```python
from build123d import *

# Parameters (mm, degrees)
BOSS_EXTRUDE1_DEPTH     = 14
SKETCH2_R               = 2.9
CUT_EXTRUDE1_DEPTH      = 48
CUT_EXTRUDE2_DEPTH      = 10
SKETCH6_R               = 10.5
CUT_EXTRUDE4_DEPTH      = 2
SKETCH8_R               = 2.9
BOSS_EXTRUDE2_DEPTH     = 4
CUT_EXTRUDE6_DEPTH      = 39.678159212
FILLET1_R               = 0.3
CUT_EXTRUDE3_DEPTH      = 4
CHAMFER1_SIZE           = 2
FILLET2_R               = 2
FILLET3_R               = 0.3
CUT_EXTRUDE5_DEPTH      = 35.583232932
CUT_EXTRUDE5_DEPTH_BACK = 35.583232932
CHAMFER2_SIZE           = 1.5


with BuildPart() as part:
    # Sketch1 → Boss-Extrude1 (new, symmetric)
    with BuildSketch(Plane(origin=(0, 0, 0), x_dir=(0, 0, -1), z_dir=(1, 0, 0))):
        with BuildLine():
            Line((30, -10), (0, -10))
            ThreePointArc((0, -10), (-10, 0), (0, 10))
            Line((0, 10), (30, 10))
            Line((30, 10), (30, -10))
        make_face()
    extrude(amount=BOSS_EXTRUDE1_DEPTH, both=True)

    # Sketch2 → Cut-Extrude1 (cut)
    with BuildSketch(Plane(origin=(14, 0, 0), x_dir=(0, 0, -1), z_dir=(1, 0, 0))):
        Circle(SKETCH2_R)
        Polygon((30, 0), (10, 10), (30, 10), align=None)
    extrude(amount=-CUT_EXTRUDE1_DEPTH, mode=Mode.SUBTRACT)

    # Sketch4 → Cut-Extrude2 (cut, symmetric)
    with BuildSketch(Plane(origin=(0, 0, 0), x_dir=(0, 0, -1), z_dir=(1, 0, 0))):
        with BuildLine():
            Line((0, -10), (4, -10))
            Line((4, -10), (4, -7.5))
            Line((4, -7.5), (10, -7.5))
            Line((10, -7.5), (15, -6))
            Line((15, -6), (30, -6))
            Line((30, -6), (30, 0))
            Line((30, 0), (10, 10))
            Line((10, 10), (0, 10))
            ThreePointArc((0, 10), (-10, 0), (0, -10))
        make_face()
    extrude(amount=CUT_EXTRUDE2_DEPTH, both=True, mode=Mode.SUBTRACT)

    # Sketch6 → Cut-Extrude4 (cut)
    with BuildSketch(Plane(origin=(-14, 0, 0), x_dir=(0, 0, -1), z_dir=(1, 0, 0))):
        Circle(SKETCH6_R)
    cut_extrude4 = extrude(amount=CUT_EXTRUDE4_DEPTH, mode=Mode.SUBTRACT)

    # Sketch8 → Boss-Extrude2 (add)
    with BuildSketch(Plane(origin=(-10, 0, 0), x_dir=(0, 0, -1), z_dir=(1, 0, 0))):
        Circle(SKETCH8_R)
    boss_extrude2 = extrude(amount=-BOSS_EXTRUDE2_DEPTH)

    # Sketch9 → Cut-Extrude6 (cut, through all)
    with BuildSketch(Plane(origin=(0, 10, 0), x_dir=(1, 0, 0), z_dir=(0, 1, 0))):
        Polygon((-14, 1), (-14, -2.9), (-12.4, -2.9), align=None)
    cut_extrude6 = extrude(amount=-CUT_EXTRUDE6_DEPTH, mode=Mode.SUBTRACT)

    # Mirror1: Cut-Extrude4, Boss-Extrude2, Cut-Extrude6 across plane
    add(cut_extrude4.mirror(Plane(origin=(0, 0, 0), x_dir=(0, 0, 1), z_dir=(1, 0, 0))), mode=Mode.SUBTRACT)
    add(boss_extrude2.mirror(Plane(origin=(0, 0, 0), x_dir=(0, 0, 1), z_dir=(1, 0, 0))))
    add(cut_extrude6.mirror(Plane(origin=(0, 0, 0), x_dir=(0, 0, 1), z_dir=(1, 0, 0))), mode=Mode.SUBTRACT)

    # Fillet1
    fillet1_edges = [part.edges().sort_by_distance(p)[0] for p in [
        (13, -10, -3.201562119),
        (13, 10, -3.201562119),
        (-13, -10, -3.201562119),
        (-13, 10, -3.201562119),
    ]]
    fillet(fillet1_edges, radius=FILLET1_R)

    # Sketch5 → Cut-Extrude3 (cut)
    with BuildSketch(Plane(origin=(0, -10, 0), x_dir=(1, 0, 0), z_dir=(0, 1, 0))):
        with BuildLine():
            Line((-3, 24.2), (3, 24.2))
            ThreePointArc((3, 24.2), (4.7, 22.5), (3, 20.8))
            Line((3, 20.8), (-3, 20.8))
            ThreePointArc((-3, 20.8), (-4.7, 22.5), (-3, 24.2))
        make_face()
    extrude(amount=CUT_EXTRUDE3_DEPTH, mode=Mode.SUBTRACT)

    # Chamfer1
    chamfer1_edges = [part.edges().sort_by_distance(p)[0] for p in [
        (0, -6, -24.2),
        (4.7, -6, -22.5),
        (0, -6, -20.8),
        (-4.7, -6, -22.5),
    ]]
    chamfer(chamfer1_edges, length=CHAMFER1_SIZE)

    # Fillet2
    fillet2_edges = [part.edges().sort_by_distance(p)[0] for p in [
        (-12, 0, -30),
        (-12, 10, -10),
        (12, 10, -10),
        (12, 0, -30),
    ]]
    fillet(fillet2_edges, radius=FILLET2_R)

    # Fillet3
    fillet3_edges = [part.edges().sort_by_distance(p)[0] for p in [
        (14, -5.618033989, -30),
        (14, 0, -10.5),
        (14, -10, -17.374342014),
        (14, -9.76770032, -4.45642273),
        (14, 9.76770032, -4.45642273),
        (-14, -10, -17.374342014),
        (-14, 0, -10.5),
        (-14, 9.76770032, -4.45642273),
        (-14, -9.76770032, -4.45642273),
        (-14, 5.170820393, -19.658359214),
        (-14, 10, -7.138274037),
        (-14, -0.184605753, -29.701301617),
        (-14, 9.946497979, -9.987369886),
        (14, 5.170820393, -19.658359214),
        (14, 10, -7.138274037),
        (14, -0.184605753, -29.701301617),
        (14, 9.946497979, -9.987369886),
        (-14, -5.618033989, -30),
    ]]
    fillet(fillet3_edges, radius=FILLET3_R)

    # Sketch7 → Cut-Extrude5 (cut, two sides: drawn at the far end of the back side and taken through both)
    with BuildSketch(Plane.ZY.offset(-CUT_EXTRUDE5_DEPTH_BACK)):
        with BuildLine():
            Line((9.767710237, 2.142857143), (6.837397166, 1.5))
            ThreePointArc((6.837397166, 1.5), (6.866578014, -1.360186158), (5.749248239, -3.993262411))
            Line((5.749248239, -3.993262411), (8.213211771, -5.704660587))
            ThreePointArc((8.213211771, -5.704660587), (9.809397162, -1.943123082), (9.767710237, 2.142857143))
        make_face()
    extrude(amount=CUT_EXTRUDE5_DEPTH + CUT_EXTRUDE5_DEPTH_BACK, mode=Mode.SUBTRACT)

    # Chamfer2
    chamfer2_edges = [part.edges().sort_by_distance(p)[0] for p in [
        (0, -7.5, -4),
    ]]
    chamfer(chamfer2_edges, length=CHAMFER2_SIZE)


solid = part.part
```
Model file for the job. Use its own axes, mm. A direction names the side the tool comes from. Round coordinates to 2 decimals unless told otherwise and drop trailing zeros. Write each loop counter-clockwise with the first axis right and the second up, starting at its lowest first coordinate (ties: lowest second). Pieces come first, ordered by that corner, then holes. Notation, with made-up numbers: (62, -33.75) -> (94, -33.75) arc R24 cw to (94, -19.75) -> close; hole circle Ø7 at (-26.5, 70). An arc over 180 degrees is marked (long way). Answer as CSV lines item,"result".
1. Slice it at A-A, the plane x = -10.75. List the corners of the cut face in (y, z).
Resolved:
outline,"(-10, -30) -> (-1.24, -30) arc R2 ccw to (0.55, -28.89) -> (9.79, -10.42) arc R2 ccw to (10, -9.53) -> (10, 0) arc R10 ccw to (2.14, 9.77) -> (1.5, 6.84) arc R7 ccw to (-3.99, 5.75) -> (-5.7, 8.21) arc R10 ccw to (-10, 0) -> close"
2. Mould opens along X. For faces 4 (the face through (13.37, 0.04, 0.54)), 5 (the face through (0, -7, -25.2)), 6 (the face through (-10.986, 1.826, 8.323)) say: +X half, -X half, draft (parallel to the pull), parting line (faces both ways), or undercut.
Resolved:
face 4,"+X half"
face 5,"undercut"
face 6,"draft"
3. Tool access for faces 1 (the face through (0, -6, -17)), 2 (the face through (-12, 2.4, -2.5)), 3 (the face through (0, -7, -19.8)): list every direction of +Z, -Z, +X, -X, +Y, -Y with a clear straight run to the whole face (end or side of a thin tool).
Resolved:
face 1,"+Z, -Z, +Y"
face 2,"-X"
face 3,"+Y"
4. Drill centre lines: line 1 (X direction, y = 6, z = 7); line 2 (X direction, y = 3, z = -20); line 3 (Z direction, x = -13, y = -0.5). Where is each one in solid material? Low to high.
Resolved:
line 1,"-12 to -10, 10 to 12"
line 2,"-14 to -10, 10 to 14"
line 3,"-29.86 to -10.49, -2.86 to 1.44"
5. Pin check, flat tips, straight feed: pin 1 Ø5 at (x, y) = (2, -3) entering from -Z; pin 2 Ø3.5 at (x, z) = (-2, -8) entering from +Y; pin 3 Ø0.5 at (x, y) = (0, -9.5) entering from +Z; pin 4 Ø10 at (x, z) = (-6.5, -17.5) entering from +Y. Stop position of each tip, or through.
Resolved:
pin 1,"through"
pin 2,"y = -7.5"
pin 3,"z = -4"
pin 4,"y = 8.04"
